Build history of the part. All positions in model axes, mm. A direction names the side the tool comes from. Round coordinates to 2 decimals unless told otherwise and drop trailing zeros. Write each loop counter-clockwise with the first axis right and the second up, starting at its lowest first coordinate (ties: lowest second). Pieces come first, ordered by that corner, then holes. Notation, with made-up numbers: M -16.5,-10 L 30.5,-10 A25 ccw 30.5,11 Z; hole C 25.5,30 d5. An arc over 180 degrees is marked long. Write item = value, one per line.
from build123d import *

# Parameters (mm, degrees)
F0_W        = 77.315364033
F0_H        = 69.4387331605
F1_DEPTH    = 50.8
F2_T        = -1.27
F3_T1_DEPTH = 109.9757379802
F3_T3_DEPTH = 102.0991071077


# Not quite as in the source:
# - a fillet or chamfer that OpenCascade refuses, or shapes differently, is made with other operations: its cross-section is extruded or revolved along the edge and cut away or added
# - the program builds the solid bodies; features that only make, move or delete a surface that nothing else refers to are left out


with BuildPart() as f1:
    # F0 (on Top) → F1 (new body)
    with BuildSketch(Plane.XY):
        with Locations((-0.1036394387, -4.8710741103)):
            Rectangle(F0_W, F0_H)
    extrude(amount=F1_DEPTH)

    # F2
    f2_openings = [f1.faces().sort_by_distance(p)[0] for p in [
        (-0.103639, -4.871074, 50.8),
    ]]
    offset(amount=F2_T, openings=f2_openings)

    # F3: chamfer of 6.35 on 4 edges, made by hand

    # F3_s2 → F3_t1 (cut)
    with BuildSketch(Plane.YZ.offset(-55.0915084288)):
        Polygon((-39.5904406905, 44.45), (-33.2404406905, 50.8), (-39.5904406905, 50.8), align=None)
        Polygon((29.84829247, 44.45), (23.49829247, 50.8), (29.84829247, 50.8), align=None)
    extrude(amount=F3_T1_DEPTH, mode=Mode.SUBTRACT)

    # F3_s4 → F3_t3 (cut)
    with BuildSketch(Plane.XZ.offset(-46.1784794436)):
        Polygon((-38.7613214552, 44.45), (-32.4113214552, 50.8), (-38.7613214552, 50.8), align=None)
        Polygon((38.5540425777, 44.45), (32.2040425777, 50.8), (38.5540425777, 50.8), align=None)
    extrude(amount=F3_T3_DEPTH, mode=Mode.SUBTRACT)


solid = f1.part
1. Tool access for faces 5 (the face through (38.554, -5, 22)), 6 (the face through (37.284, -5, 23)): list every direction of +Z, -Z, +X, -X, +Y, -Y with a clear straight run to the whole face (end or side of a thin tool).
Responses:
face_5 = +Z, -Z, +X, +Y, -Y
face_6 = +Z
2. Band-saw the part on A-A (z = 38). List the corners of the cut face in (x, y).
Responses:
outline = M -38.76,-39.59 L 38.55,-39.59 L 38.55,29.85 L -38.76,29.85 Z; hole M -37.49,-38.32 L 37.28,-38.32 L 37.28,28.58 L -37.49,28.58 Z
3. Band-saw the part on B-B (x = 23). List the corners of the cut face in (y, z).
Responses:
outline = M -39.59,0 L 29.85,0 L 29.85,44.45 L 28.58,45.72 L 28.58,1.27 L -38.32,1.27 L -38.32,45.72 L -39.59,44.45 Z
4. Flat gauge pins, fed straight in: pin 1 (12 mm diameter, centred on x = 27, y = -15, fed in from -Z); pin 2 (4 mm diameter, centred on x = -0.5, y = 0, fed in from +Z). Where does each tip first touch, or does it go through?
Responses:
pin_1 = 0
pin_2 = 1.27
5. Band-saw the part on C-C (y = 12). List the corners of the cut face in (x, z), plus the area to 3 significant figures.
Responses:
outline = M -38.76,0 L 38.55,0 L 38.55,44.45 L 37.28,45.72 L 37.28,1.27 L -37.49,1.27 L -37.49,45.72 L -38.76,44.45 Z
area = 209 mm²
6. Mould opens along Y. For faces 1 (the face through (-1, 29.848, 22)), 2 (the face through (-1, -4, 0)), 3 (the face through (-37.491, -5, 23)), 4 (the face through (-1, -39.59, 22)) say: pulls with the +Y half, pulls with the -Y half, needs draft (parallel to the pull), parting line crosses it, or undercut.
Responses:
face_1 = pulls with the +Y half
face_2 = needs draft
face_3 = undercut
face_4 = pulls with the -Y half
7. Probe probe 1 along Y at (x, z) = (15.5, 31.5); probe 2 along X at (y, z) = (15.5, 25.5); probe 3 along Z at (x, y) = (-18, -13.5). List the from-to ranges inside material, lowest first.
Responses:
probe_1 = -39.59 to -38.32, 28.58 to 29.85
probe_2 = -38.76 to -37.49, 37.28 to 38.55
probe_3 = 0 to 1.27
